```python
from build123d import *

# Parameters (mm, degrees)
SKETCH2_W                                  = 25
SKETCH2_H                                  = 25
BOSS_EXTRUDE1_MODULE_PCB_DEPTH             = 1.6
FILLET1_CORNERS_R                          = 2.5
SKETCH3_R                                  = 1.55
CUT_EXTRUDE1_FIRST_MH_DEPTH                = 1.6
SKETCH4_R                                  = 2.2
SKETCH4_R_2                                = 1.55
BOSS_EXTRUDE2_PTH_FOR_FIRST_MH_DEPTH       = 0.01
MIRROR2_SECOND_MH_PTH_COPY_1_SKETCH_R      = 2.2
MIRROR2_SECOND_MH_PTH_COPY_1_SKETCH_R_2    = 1.55
MIRROR2_SECOND_MH_PTH_COPY_1_DEPTH         = 0.01
MIRROR3_REMAINING_MH_PTH_COPY_1_SKETC_R    = 1.55
MIRROR3_REMAINING_MH_PTH_COPY_1_DEPTH      = 1.6
MIRROR3_REMAINING_MH_PTH_COPY_2_SKETC_R    = 2.2
MIRROR3_REMAINING_MH_PTH_COPY_2_SKETC_R_2  = 1.55
MIRROR3_REMAINING_MH_PTH_COPY_2_DEPTH      = 0.01
MIRROR3_REMAINING_MH_PTH_COPY_3_SKETC_R    = 2.2
MIRROR3_REMAINING_MH_PTH_COPY_3_SKETC_R_2  = 1.55
MIRROR3_REMAINING_MH_PTH_COPY_3_DEPTH      = 0.01
MIRROR3_REMAINING_MH_PTH_COPY_4_SKETC_R    = 2.2
MIRROR3_REMAINING_MH_PTH_COPY_4_SKETC_R_2  = 1.55
MIRROR3_REMAINING_MH_PTH_COPY_4_DEPTH      = 0.01
BOSS_EXTRUDE1_REACH                        = 3.62
SKETCH5_W                                  = 6.54
SKETCH5_H                                  = 1.6
BOSS_EXTRUDE3_TIP_OF_EDGE_CONNECTOR_DEPTH  = 1.5
SKETCH6_W                                  = 2.7
SKETCH6_H                                  = 1.6
CUT_EXTRUDE2_SIDES_OF_EDGE_CONNECTOR_DEPTH = 4.35
FILLET2_TIP_OF_EDGE_CONNECTOR_R            = 0.8
FILLET3_BASE_OF_EDGE_CONNECTOR_R           = 1
FILLET4_ADJACENT_TO_EDGE_CONNECTOR_R       = 0.8


with BuildPart() as part:
    # Sketch2 → Boss-Extrude1 _module PCB (new body)
    with BuildSketch(Plane.XY):
        Rectangle(SKETCH2_W, SKETCH2_H)
    extrude(amount=BOSS_EXTRUDE1_MODULE_PCB_DEPTH)

    # Fillet1 _corners
    fillet1_corners_edges = [part.edges().sort_by_distance(p)[0] for p in [
        (12.5, -12.5, 0.8),
        (-12.5, -12.5, 0.8),
        (-12.5, 12.5, 0.8),
        (12.5, 12.5, 0.8),
    ]]
    fillet(fillet1_corners_edges, radius=FILLET1_CORNERS_R)

    # Sketch3 → Cut-Extrude1 _first MH (cut)
    with BuildSketch(Plane.XY):
        with Locations((10, 10)):
            Circle(SKETCH3_R)
    cut_extrude1_first_mh = extrude(amount=CUT_EXTRUDE1_FIRST_MH_DEPTH, mode=Mode.SUBTRACT)

    # Sketch4 → Boss-Extrude2 _PTH for first MH (add)
    with BuildSketch(Plane.XY):
        with Locations((10, 10)):
            Circle(SKETCH4_R)
        with Locations((10, 10)):
            Circle(SKETCH4_R_2, mode=Mode.SUBTRACT)
    boss_extrude2_pth_for_first_mh = extrude(amount=-BOSS_EXTRUDE2_PTH_FOR_FIRST_MH_DEPTH)

    # Mirror1 _PTH for first MH: Boss-Extrude2 _PTH for first MH across plane
    add(boss_extrude2_pth_for_first_mh.mirror(Plane.XY.offset(0.8)))

    # Mirror2 _second MH _ PTH: Cut-Extrude1 _first MH, Boss-Extrude2 _PTH for first MH across plane
    add(cut_extrude1_first_mh.mirror(Plane(origin=(0, 0, 0), x_dir=(0, 0, 1), z_dir=(1, 0, 0))), mode=Mode.SUBTRACT)
    add(boss_extrude2_pth_for_first_mh.mirror(Plane(origin=(0, 0, 0), x_dir=(0, 0, 1), z_dir=(1, 0, 0))))

    # Mirror2 _second MH _ PTH copy 1 sketch → Mirror2 _second MH _ PTH copy 1 (add)
    with BuildSketch(Plane(origin=(0, 0, 1.6), x_dir=(-1, 0, 0), z_dir=(0, 0, -1))):
        with Locations((10, 10)):
            Circle(MIRROR2_SECOND_MH_PTH_COPY_1_SKETCH_R)
        with Locations((10, 10)):
            Circle(MIRROR2_SECOND_MH_PTH_COPY_1_SKETCH_R_2, mode=Mode.SUBTRACT)
    extrude(amount=-MIRROR2_SECOND_MH_PTH_COPY_1_DEPTH)

    # Mirror3 _remaining MH _ PTH: Cut-Extrude1 _first MH, Boss-Extrude2 _PTH for first MH across plane
    add(cut_extrude1_first_mh.mirror(Plane.ZX), mode=Mode.SUBTRACT)
    add(boss_extrude2_pth_for_first_mh.mirror(Plane.ZX))

    # Mirror3 _remaining MH _ PTH copy 1 sketc → Mirror3 _remaining MH _ PTH copy 1 (cut)
    with BuildSketch(Plane(origin=(0, 0, 0), x_dir=(-1, 0, 0), z_dir=(0, 0, 1))):
        with Locations((10, 10)):
            Circle(MIRROR3_REMAINING_MH_PTH_COPY_1_SKETC_R)
    extrude(amount=MIRROR3_REMAINING_MH_PTH_COPY_1_DEPTH, mode=Mode.SUBTRACT)

    # Mirror3 _remaining MH _ PTH copy 2 sketc → Mirror3 _remaining MH _ PTH copy 2 (add)
    with BuildSketch(Plane(origin=(0, 0, 0), x_dir=(-1, 0, 0), z_dir=(0, 0, 1))):
        with Locations((10, 10)):
            Circle(MIRROR3_REMAINING_MH_PTH_COPY_2_SKETC_R)
        with Locations((10, 10)):
            Circle(MIRROR3_REMAINING_MH_PTH_COPY_2_SKETC_R_2, mode=Mode.SUBTRACT)
    extrude(amount=-MIRROR3_REMAINING_MH_PTH_COPY_2_DEPTH)

    # Mirror3 _remaining MH _ PTH copy 3 sketc → Mirror3 _remaining MH _ PTH copy 3 (add)
    with BuildSketch(Plane(origin=(0, 0, 1.6), x_dir=(-1, 0, 0), z_dir=(0, 0, -1))):
        with Locations((10, -10)):
            Circle(MIRROR3_REMAINING_MH_PTH_COPY_3_SKETC_R)
        with Locations((10, -10)):
            Circle(MIRROR3_REMAINING_MH_PTH_COPY_3_SKETC_R_2, mode=Mode.SUBTRACT)
    extrude(amount=-MIRROR3_REMAINING_MH_PTH_COPY_3_DEPTH)

    # Mirror3 _remaining MH _ PTH copy 4 sketc → Mirror3 _remaining MH _ PTH copy 4 (add)
    with BuildSketch(Plane(origin=(0, 0, 1.6), x_dir=(1, 0, 0), z_dir=(0, 0, -1))):
        with Locations((10, 10)):
            Circle(MIRROR3_REMAINING_MH_PTH_COPY_4_SKETC_R)
        with Locations((10, 10)):
            Circle(MIRROR3_REMAINING_MH_PTH_COPY_4_SKETC_R_2, mode=Mode.SUBTRACT)
    extrude(amount=-MIRROR3_REMAINING_MH_PTH_COPY_4_DEPTH)

    # Sketch7 → Boss-Extrude1 (add, up to next)
    with BuildSketch(Plane(origin=(0, 0, -0.01), x_dir=(-1, 0, 0), z_dir=(0, 0, -1)), mode=Mode.PRIVATE) as boss_extrude1_sk1:
        with BuildLine():
            Line((-10, -7.8), (-12.2, -7.8))
            Line((-12.2, -7.8), (-12.2, -10))
            ThreePointArc((-12.2, -10), (-11.555634919, -8.444365081), (-10, -7.8))
        make_face()
    boss_extrude1_tool1 = extrude(boss_extrude1_sk1.sketch, amount=-BOSS_EXTRUDE1_REACH, mode=Mode.PRIVATE) - part.part
    add(boss_extrude1_tool1.solids().sort_by_distance((11.708591, -8.291409, -0.01))[0])
    # Sketch7 → Boss-Extrude1 (add, up to next)
    with BuildSketch(Plane(origin=(0, 0, -0.01), x_dir=(-1, 0, 0), z_dir=(0, 0, -1)), mode=Mode.PRIVATE) as boss_extrude1_sk2:
        with BuildLine():
            Line((-10, -12.2), (-7.8, -12.2))
            Line((-7.8, -12.2), (-7.8, -10))
            ThreePointArc((-7.8, -10), (-8.444365081, -11.555634919), (-10, -12.2))
        make_face()
    boss_extrude1_tool2 = extrude(boss_extrude1_sk2.sketch, amount=-BOSS_EXTRUDE1_REACH, mode=Mode.PRIVATE) - part.part
    add(boss_extrude1_tool2.solids().sort_by_distance((8.291409, -11.708591, -0.01))[0])

    # Sketch5 → Boss-Extrude3 _tip of edge connector (add)
    with BuildSketch(Plane(origin=(0, 12.5, 0), x_dir=(1, 0, 0), z_dir=(0, 1, 0))):
        with Locations((0, -0.8)):
            Rectangle(SKETCH5_W, SKETCH5_H)
    extrude(amount=BOSS_EXTRUDE3_TIP_OF_EDGE_CONNECTOR_DEPTH)

    # Sketch6 → Cut-Extrude2 _sides of edge connector (cut)
    with BuildSketch(Plane(origin=(0, 12.5, 0), x_dir=(1, 0, 0), z_dir=(0, 1, 0))):
        with Locations((-4.62, -0.8)):
            Rectangle(SKETCH6_W, SKETCH6_H)
        with Locations((4.62, -0.8)):
            Rectangle(SKETCH6_W, SKETCH6_H)
    extrude(amount=-CUT_EXTRUDE2_SIDES_OF_EDGE_CONNECTOR_DEPTH, mode=Mode.SUBTRACT)

    # Fillet2 _tip of edge connector
    fillet2_tip_of_edge_connector_edges = [part.edges().sort_by_distance(p)[0] for p in [
        (3.27, 14, 0.8),
        (-3.27, 14, 0.8),
    ]]
    fillet(fillet2_tip_of_edge_connector_edges, radius=FILLET2_TIP_OF_EDGE_CONNECTOR_R)

    # Fillet3 _base of edge connector
    fillet3_base_of_edge_connector_edges = [part.edges().sort_by_distance(p)[0] for p in [
        (-3.27, 8.15, 0.8),
        (-5.97, 8.15, 0.8),
        (3.27, 8.15, 0.8),
        (5.97, 8.15, 0.8),
    ]]
    fillet(fillet3_base_of_edge_connector_edges, radius=FILLET3_BASE_OF_EDGE_CONNECTOR_R)

    # Fillet4 _adjacent to edge connector
    fillet4_adjacent_to_edge_connector_edges = [part.edges().sort_by_distance(p)[0] for p in [
        (-5.97, 12.5, 0.8),
        (5.97, 12.5, 0.8),
    ]]
    fillet(fillet4_adjacent_to_edge_connector_edges, radius=FILLET4_ADJACENT_TO_EDGE_CONNECTOR_R)


solid = part.part
```
Model file for the job. Use its own axes, mm. A direction names the side the tool comes from. Give positions to 0.01 mm unless a question says otherwise; leave off trailing zeros. Write each loop counter-clockwise with the first axis right and the second up, starting at its lowest first coordinate (ties: lowest second). Pieces come first, ordered by that corner, then holes. Notation, with made-up numbers: (-8, 73.25) -> (42, 73.25) arc R19 ccw to (42, 93.25) -> close; hole circle Ø2 at (86, 82.5). An arc over 180 degrees is marked (long way). Use CSV: the item, a comma, the result in double quotes. Start each with the question number.
1) Cut at A-A on z = 0.85. List the corners of the cut face in (x, y), plus the area to 3 significant figures.
2) Two-plate mould, pull along X, no slides. Class faces 4 (the flat face through (12.5, 0, 1)), 5 (the cylindrical face through (3.555, 8.451, 0.789)), 6 (the flat face through (-10.95, 8.56, 1.61)), 7 (the flat face through (-3.27, 11, 1)): released by +X, released by -X, zero draft, split by the parting line, or undercut.
3) Drill centre lines: L1, parallel to X at y = -10, z = 0.75; L2, parallel to X at y = -8.75, z = 0.25. Where is each one in solid material? Low to high.
4) Cut at B-B on y = -9.5. Count the separate pieces of the cut face and the enclosed holes in it, plus the area to 3 significant figures.
5) Tool access for faces 1 (the cylindrical face through (6.2, 12.26, 0.79)), 2 (the flat face through (0, -12.5, 1)), 3 (the flat face through (8, 12.5, 1)): list every direction of +Z, -Z, +X, -X, +Y, -Y with a clear straight run to the whole face (end or side of a thin tool).
6) Pin check, flat tips, straight feed: P1, Ø12, axis at x = 5, y = 10, coming from the -Z side; P2, Ø0.5, axis at y = 11.5, z = 0.5, coming from the -X side; P3, Ø8, axis at x = 8, y = -0.5, coming from the +Z side; P4, Ø0.5, axis at x = 9, z = 1, coming from the +Y side. Stop position of each tip, or through.
Final values:
1,outline,"(-12.5, -10) arc R2.5 ccw to (-10, -12.5) -> (10, -12.5) arc R2.5 ccw to (12.5, -10) -> (12.5, 10) arc R2.5 ccw to (10, 12.5) -> (6.77, 12.5) arc R0.8 ccw to (5.97, 11.7) -> (5.97, 9.15) arc R1 cw to (4.97, 8.15) -> (4.27, 8.15) arc R1 cw to (3.27, 9.15) -> (3.27, 13.2) arc R0.8 ccw to (2.47, 14) -> (-2.47, 14) arc R0.8 ccw to (-3.27, 13.2) -> (-3.27, 9.15) arc R1 cw to (-4.27, 8.15) -> (-4.97, 8.15) arc R1 cw to (-5.97, 9.15) -> (-5.97, 11.7) arc R0.8 ccw to (-6.77, 12.5) -> (-10, 12.5) arc R2.5 ccw to (-12.5, 10) -> close; hole circle Ø3.1 at (-10, -10); hole circle Ø3.1 at (-10, 10); hole circle Ø3.1 at (10, -10); hole circle Ø3.1 at (10, 10)"
1,area,"576 mm2"
2,face 4,"released by +X"
2,face 5,"undercut"
2,face 6,"zero draft"
2,face 7,"undercut"
3,L1,"x = -12.5 to -11.55, -8.45 to 8.45, 11.55 to 12.5"
3,L2,"x = -12.5 to -10.92, -9.08 to 9.08, 10.92 to 12.5"
4,separate pieces,"3"
4,enclosed holes,"0"
4,area,"30.7 mm2"
5,face 1,"+Z, -Z, +Y"
5,face 2,"+Z, -Z, +X, -X, -Y"
5,face 3,"+Z, -Z, +X, +Y"
6,P1,"stops at z = -0.01"
6,P2,"stops at x = -12.17"
6,P3,"stops at z = 1.6"
6,P4,"stops at y = 12.5"
